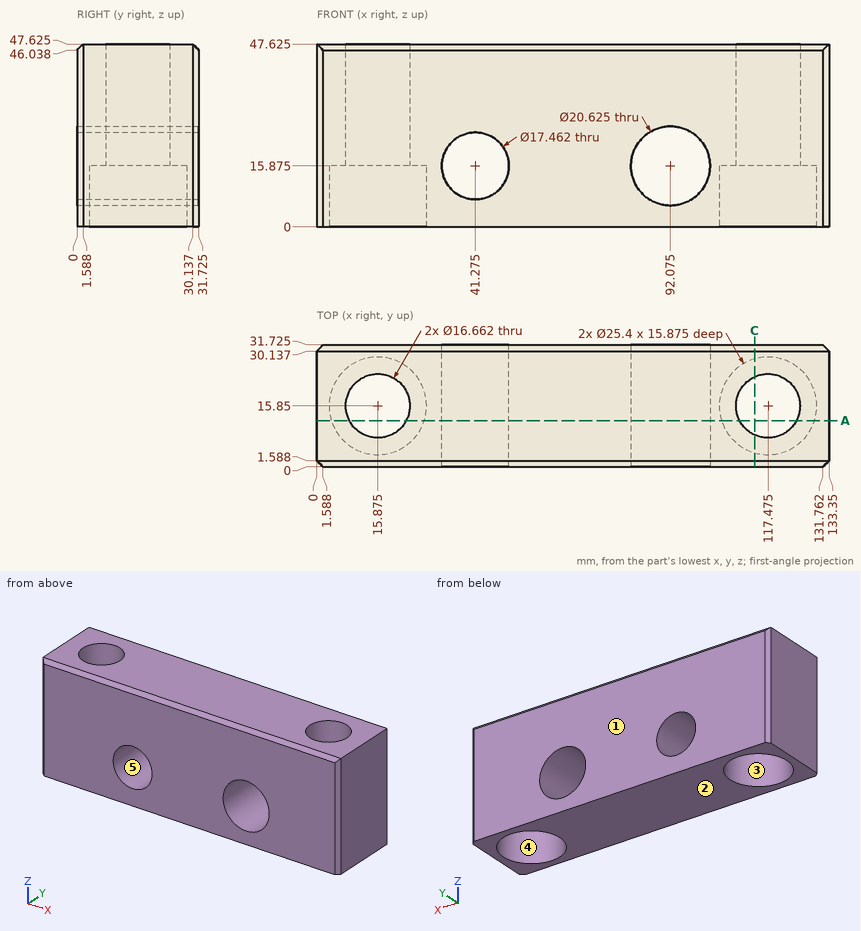
Source: three-view drawing plus pictorial views. Frame: mm from the lowest corner of the part. A direction names the side the tool comes from. Round coordinates to 2 decimals unless told otherwise and drop trailing zeros. Loops run counter-clockwise (first coordinate to the right, second up) from the corner with the lowest first, then second, coordinate; pieces in that order, holes last.
Q1. First-contact query: P1, Ø19, axis at x = 117.48, y = 15.85, coming from the -Z side (1 decimal). Flat tip, straight axial feed; report the tip coordinate or a pass-through.
Q2. Section C-C, the plane x = 114. Return loops of the section in (y, z) (1 decimal).
Q3. Mould query, pull axis Y, two halves, no side actions, for the marked faces 1, 2 and 3. Classes: pulls with the +Y half, pulls with the -Y half, needs draft (parallel to the pull), parting line crosses it, or undercut.
Q4. Section A-A, the plane y = 12. State how many separate pieces and enclosed holes the cut face has, plus the area to 3 significant figures.
Q5. Ray query, line 1 (X direction, y = 20, z = 31); line 2 (X direction, y = 14, z = 45); line 3 (Z direction, x = 23, y = 11) (1 decimal). Return the intervals inside material, ascending.
Q6. Access query for the marked faces 4 and 5. Directions: +Z, -Z, +X, -X, +Y, -Y. A direction counts if a zero-diameter tool reaches every point of the face in a straight line with its end or side. Return the directions, or none.
Solutions:
1. P1: stops at z = 15.9
2. outline: (0, 0) - (3.6, 0) - (3.6, 15.9) - (8.3, 15.9) - (8.3, 47.6) - (1.6, 47.6) - (0, 46) - close; (23.4, 15.9) - (28.1, 15.9) - (28.1, 0) - (31.7, 0) - (31.7, 46) - (30.1, 47.6) - (23.4, 47.6) - close
3. face 1: pulls with the +Y half
3. face 2: needs draft
3. face 3: undercut
4. separate pieces: 3
4. enclosed holes: 2
4. area: 4,070 mm2
5. line 1: x = 0 to 8.65, 23.1 to 110.25, 124.7 to 133.35
5. line 2: x = 0 to 7.75, 24 to 109.35, 125.6 to 133.35
5. line 3: z = 15.9 to 47.6
6. face 4: -Z
6. face 5: +Y, -Y
